```python
from build123d import *

# Parameters (mm, degrees)
F0_R     = 5
F1_DEPTH = 250
F2_R     = 1


with BuildPart() as f1:
    # F0 (on Front) → F1 (new body, symmetric)
    with BuildSketch(Plane.XZ):
        Polygon((20, 5), (20, 20), (5, 20), (5, 14), (10.05, 14), (10.05, 11.5), (6.05, 7.5), (-6.05, 7.5), (-10.05, 11.5), (-10.05, 14), (-5, 14), (-5, 20), (-20, 20), (-20, 5), (-14, 5), (-14, 10.05), (-11.5, 10.05), (-7.5, 6.05), (-7.5, -6.05), (-11.5, -10.05), (-14, -10.05), (-14, -5), (-20, -5), (-20, -20), (-5, -20), (-5, -14), (-10.05, -14), (-10.05, -11.5), (-6.05, -7.5), (6.05, -7.5), (10.05, -11.5), (10.05, -14), (5, -14), (5, -20), (20, -20), (20, -5), (14, -5), (14, -10.05), (11.5, -10.05), (7.5, -6.05), (7.5, 6.05), (11.5, 10.05), (14, 10.05), (14, 5), align=None)
        Circle(F0_R, mode=Mode.SUBTRACT)
    extrude(amount=F1_DEPTH, both=True)

    # F2
    f2_edges = [f1.edges().sort_by_distance(p)[0] for p in [
        (-5, 0, 20),
        (5, 0, 20),
        (20, 0, 20),
        (20, 0, 5),
        (-5, 0, 14),
        (-6.05, 0, 7.5),
        (-10.05, 0, 11.5),
        (-10.05, 0, 14),
        (10.05, 0, 14),
        (5, 0, 14),
        (10.05, 0, 11.5),
        (6.05, 0, 7.5),
        (20, 0, -5),
        (14, 0, -5),
        (7.5, 0, 6.05),
        (7.5, 0, -6.05),
        (-10.05, 0, -11.5),
        (-10.05, 0, -14),
        (5, 0, -14),
        (20, 0, -20),
        (-5, 0, -20),
        (-14, 0, -5),
        (-14, 0, -10.05),
        (-14, 0, 5),
        (-20, 0, 20),
        (14, 0, -10.05),
        (10.05, 0, -11.5),
        (10.05, 0, -14),
        (-5, 0, -14),
        (5, 0, -20),
        (-14, 0, 10.05),
        (-20, 0, 5),
        (-20, 0, -5),
        (-7.5, 0, 6.05),
        (-7.5, 0, -6.05),
        (-11.5, 0, -10.05),
        (14, 0, 10.05),
        (11.5, 0, 10.05),
        (14, 0, 5),
        (-6.05, 0, -7.5),
        (6.05, 0, -7.5),
        (-20, 0, -20),
    ]]
    fillet(f2_edges, radius=F2_R)


solid = f1.part
```
Here's how the part is built. I have some questions about the finished solid (model axes, mm). Give positions to 0.01 mm unless a question says otherwise; leave off trailing zeros. Write each loop counter-clockwise with the first axis right and the second up, starting at its lowest first coordinate (ties: lowest second). Pieces come first, ordered by that corner, then holes.
(1) Will these pins go through, and if not, where does the flat tip stop? pin 1 (6 mm diameter, centred on x = -2.5, y = -144, fed in from -Z); pin 2 (5.5 mm diameter, centred on y = -32, z = 2.5, fed in from +X); pin 3 (8 mm diameter, centred on x = 0, z = 0, fed in from -Y).
Output values:
pin 1: stops at z = -19.87
pin 2: stops at x = 19.66
pin 3: passes through
(2) Imagine slicing it at A-A, the plane z = 0. Write out the boundary of the cut face in (x, y), and give its area (3 significant figures).
Output values:
outline: (-7.5, -250) - (-5, -250) - (-5, 250) - (-7.5, 250) - close; (5, -250) - (7.5, -250) - (7.5, 250) - (5, 250) - close
area: 2,500 mm2
(3) If I drill on L1, parallel to Z at x = 0, y = -112; L2, parallel to X at y = 196.5, z = -17.5; L3, parallel to Z at x = 1, y = -212, over which ranges is the centre line in solid material (lowest first)?
Output values:
L1: z = -7.5 to -5, 5 to 7.5
L2: x = -20 to -5, 5 to 20
L3: z = -7.5 to -4.9, 4.9 to 7.5
(4) Thinking about a two-plate mould opening in X: for faces 1 (the face through (0, -4, 7.5)), 2 (the face through (-5, 250, -4)), 3 (the face through (-20, -4, -12)), 4 (the face through (20, -4, -13)), which applies, pulls with the +X half, pulls with the -X half, needs draft (parallel to the pull), parting line crosses it, or undercut?
Output values:
face 1: undercut
face 2: needs draft
face 3: pulls with the -X half
face 4: pulls with the +X half
(5) Imagine slicing it at B-B, the plane x = 0. Write out the boundary of the cut face in (y, z), and give its area (3 significant figures).
Output values:
outline: (-250, -7.5) - (250, -7.5) - (250, -5) - (-250, -5) - close; (-250, 5) - (250, 5) - (250, 7.5) - (-250, 7.5) - close
area: 2,500 mm2
